Could you check a few things on this model? Use its own coordinates, in mm. Round coordinates to 2 decimals unless told otherwise and drop trailing zeros. Write each loop counter-clockwise with the first axis right and the second up, starting at its lowest first coordinate (ties: lowest second). Pieces come first, ordered by that corner, then holes. Notation, with made-up numbers: (75, -14) - (94, -14) arc R22 ccw to (94, 15) - close; hole circle Ø8 at (72.5, 79.25). An arc over 180 degrees is marked (long way). Put each result on its own line as item: value.
from build123d import *

# Parameters (mm, degrees)
F1_DEPTH      = 33.5
F1_DEPTH_BACK = 10


with BuildPart() as f1:
    # F0 (on Right) → F1 (new body, two sides)
    with BuildSketch(Plane.YZ) as f1_sk:
        Polygon((0, -62.5), (0, 0), (5, 0), (5, -2), (8, -2), (8, 4), (-5, 4), (-5, -67.5), (10, -67.5), (10, -62.5), align=None)
    extrude(amount=F1_DEPTH)
    extrude(f1_sk.sketch, amount=-F1_DEPTH_BACK)


solid = f1.part
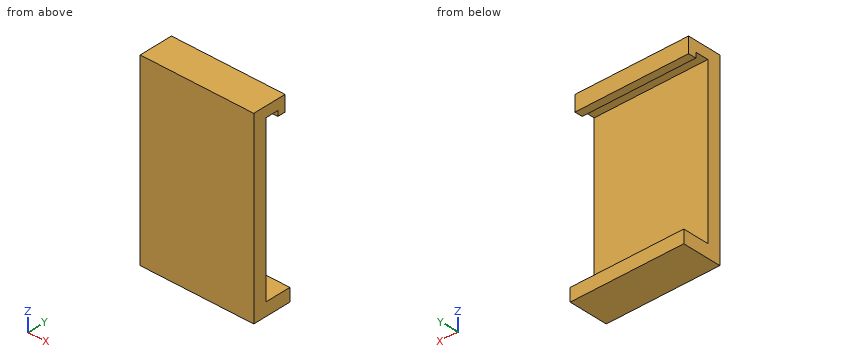
(1) Please list where these lines run through material, in increasing order: probe 1 along Z at (x, y) = (30.5, 1); probe 2 along Z at (x, y) = (-2.5, 6.5); probe 3 along Y at (x, z) = (-6, -60.5). Write a range as from..to.
Values found:
probe 1: z = -67.5..-62.5, 0..4
probe 2: z = -67.5..-62.5, -2..4
probe 3: y = -5..0
(2) I'm going to push flat-ended pins straight in: pin 1 (5 mm diameter, centred on x = 9.5, z = -44, fed in from +Y); pin 2 (1.8 mm diameter, centred on x = 3.5, z = 1, fed in from +Y); pin 3 (4 mm diameter, centred on y = 3.5, z = -60, fed in from +X) (1 decimal). Where does each tip first touch, or does it pass through?
Values found:
pin 1: stops at y = 0
pin 2: stops at y = 8
pin 3: passes through
(3) Imagine slicing it at A-A, the plane x = 20.5. List the corners of the cut face in (y, z) for me, then the cut area to 4 significant figures.
Values found:
outline: (-5, -67.5) - (10, -67.5) - (10, -62.5) - (0, -62.5) - (0, 0) - (5, 0) - (5, -2) - (8, -2) - (8, 4) - (-5, 4) - close
area: 445.5 mm^2
(4) Imagine slicing it at B-B, the plane y = 9. List the corners of the cut face in (x, z) for me.
Values found:
outline: (-10, -67.5) - (33.5, -67.5) - (33.5, -62.5) - (-10, -62.5) - close
(5) Imagine slicing it at C-C, the plane z = -60.5. List the corners of the cut face in (x, y) for me, then the cut area to 4 significant figures.
Values found:
outline: (-10, -5) - (33.5, -5) - (33.5, 0) - (-10, 0) - close
area: 217.5 mm^2
